Geometry: final body of the model. Coordinates: model frame, mm. A direction names the side the tool comes from. Give positions to 0.01 mm unless a question says otherwise; leave off trailing zeros. Write each loop counter-clockwise with the first axis right and the second up, starting at its lowest first coordinate (ties: lowest second). Pieces come first, ordered by that corner, then holes. Notation, with made-up numbers: M 78.25,28 L 133.25,28 A22 ccw 133.25,53 Z; hole C 69.25,-16.5 d9. An arc over 180 degrees is marked long. Use a Markdown table: item, result. Add a question column.
1) Pin query (flat end, axial travel): pin 1 (0.9 mm diameter, centred on x = 59, z = 5, fed in from +Y); pin 2 (2.5 mm diameter, centred on x = 29.5, y = 31, fed in from -Z); pin 3 (1 mm diameter, centred on x = -60.5, z = 1, fed in from -Y); pin 4 (2.5 mm diameter, centred on x = 56.5, z = 4.5, fed in from -Y). Return the tip coordinate at first contact, or that it passes through.
2) Section D-D on z = 4. State how many separate pieces and enclosed holes the cut face has, then the cut area to 3 significant figures.
3) Section A-A on y = 9. Return the cut outline in (x, z) (3 decimals), then the cut area to 3 significant figures.
4) Section B-B on y = 1. Return the cut outline in (x, z) (3 decimals).
5) Line query: line 1 (X direction, y = 5.5, z = 4.75) (3 decimals); line 2 (X direction, y = 29, z = 2.25) (3 decimals); line 3 (Z direction, x = 22, y = 11.5). Output: solid intervals per line, ascending.
6) Set-up query: faces 1 (the flat face through (13, 30, 2.75)), 2 (the flat face through (14.531, 12.6, 2.6)), 3 (the flat face through (21.175, 28, 4)). Return all of +Z, -Z, +X, -X, +Y, -Y with unobstructed straight access to the full face (end or side cutting, diameter ignored); none if empty.
7) Section C-C on x = 26.5. Return the cut outline in (y, z), then the cut area to 3 significant figures.
8) Draft query along X for faces 4 (the flat face through (46, 30, 2.75)), 5 (the flat face through (19, 4.871, 4)), 6 (the flat face through (62.175, -11.7, 2.6)). Return one class per face: +X half, -X half, draft (parallel to the pull), parting line (faces both ways), or undercut.
```python
from build123d import *

# Parameters (mm, degrees)
F0_R          = 2.5
F1_DEPTH      = 2
F3_R          = 0.99999
F2_W          = 15.5
F2_H          = 9
F2_W_2        = 9
F2_H_2        = 15.5
F2_W_3        = 37
F2_H_3        = 37
F4_DEPTH      = 0.5
F5_DEPTH      = 0.5
F6_DEPTH      = 5
F7_W          = 14
F7_H          = 3
F8_DEPTH      = 107.3565227488
F8_DEPTH_BACK = 60.2954772512
F9_W          = 13
F9_H          = 3
F10_DEPTH     = 5
F11_DEPTH     = 4


# Not quite as in the source:
# - a fillet or chamfer is up to 0.001 mm smaller than in the source, because OpenCascade refuses the exact size


with BuildPart() as f1:
    # F0 (on Top) → F1 (new body)
    with BuildSketch(Plane.XY):
        Polygon((83.825, -24.3705166107), (83.825, 32.3705166107), (-83.825, 32.3705166107), (-83.825, -32.3705166107), (-68.825, -32.3705166107), (-68.825, -24.3705166107), (-50.825, -24.3705166107), (-50.825, -32.3705166107), (-42.825, -32.3705166107), (-42.825, -24.3705166107), (-38.825, -24.3705166107), (-38.825, -36.5294833893), (-27.825, -36.5294833893), (-27.825, -28.5294833893), (-25.825, -28.5294833893), (-25.825, -36.5294833893), (45.175, -36.5294833893), (45.175, -24.3705166107), align=None)
        with Locations((-76.325, -27.6294833893)):
            Circle(F0_R, mode=Mode.SUBTRACT)
        with Locations((-76.325, 15.8705166107)):
            Circle(F0_R, mode=Mode.SUBTRACT)
    extrude(amount=F1_DEPTH)

    # F3 (radius 1 in the source; OpenCascade refuses exactly that, so slightly less here)
    f3_edges = [f1.edges().sort_by_distance(p)[0] for p in [
        (-83.825, -32.370517, 1),
        (-68.825, -32.370517, 1),
        (-68.825, -24.370517, 1),
        (-50.825, -32.370517, 1),
        (-42.825, -32.370517, 1),
        (-42.825, -24.370517, 1),
        (-38.825, -36.529483, 1),
        (-27.825, -36.529483, 1),
        (-27.825, -28.529483, 1),
        (-25.825, -36.529483, 1),
        (83.825, -24.370517, 1),
        (45.175, -24.370517, 1),
        (45.175, -36.529483, 1),
        (83.825, 32.370517, 1),
        (-83.825, 32.370517, 1),
        (-50.825, -24.370517, 1),
        (-38.825, -24.370517, 1),
        (-25.825, -28.529483, 1),
    ]]
    fillet(f3_edges, radius=F3_R)

    # F2 (on face) → F4 (cut)
    with BuildSketch(Plane.XY.offset(2)):
        with Locations((-70.075, 27.8705166107)):
            Rectangle(F2_W, F2_H)
        with Locations((-53.575, 27.8705166107)):
            Rectangle(F2_W, F2_H)
        with Locations((-37.075, 27.8705166107)):
            Rectangle(F2_W, F2_H)
        with Locations((-20.575, 27.8705166107)):
            Rectangle(F2_W, F2_H)
        with Locations((-4.075, 27.8705166107)):
            Rectangle(F2_W, F2_H)
        with Locations((12.425, 27.8705166107)):
            Rectangle(F2_W, F2_H)
        with Locations((28.925, 27.8705166107)):
            Rectangle(F2_W, F2_H)
        with Locations((45.425, 27.8705166107)):
            Rectangle(F2_W, F2_H)
        with Locations((61.925, 27.8705166107)):
            Rectangle(F2_W, F2_H)
        with Locations((57.675, 12.6205166107)):
            Rectangle(F2_W_2, F2_H_2)
        with Locations((57.675, -11.6205166107)):
            Rectangle(F2_W_2, F2_H_2)
        with Locations((19.0305227488, 12.6205166107)):
            Rectangle(F2_W_2, F2_H_2)
        with Locations((19.0305227488, -11.6205166107)):
            Rectangle(F2_W_2, F2_H_2)
        with Locations((-33.1395904124, -0.086670503)):
            Rectangle(F2_W_3, F2_H_3)
    extrude(amount=-F4_DEPTH, mode=Mode.SUBTRACT)

    # F5 (add, through all): faces of the model
    f5_faces = [f1.faces().sort_by_distance(p)[0] for p in [
        (-70.075, 27.8705166107, 1.5),
        (-53.575, 27.8705166107, 1.5),
        (-37.075, 27.8705166107, 1.5),
        (-20.575, 27.8705166107, 1.5),
        (-4.075, 27.8705166107, 1.5),
    ]]
    extrude(f5_faces, amount=F5_DEPTH)

    # F6 (add): faces of the model
    f6_faces = [f1.faces().sort_by_distance(p)[0] for p in [
        (12.425, 27.8705166107, 1.5),
        (28.925, 27.8705166107, 1.5),
        (45.425, 27.8705166107, 1.5),
        (61.925, 27.8705166107, 1.5),
        (19.0305227488, 12.6205166107, 1.5),
        (57.675, 12.6205166107, 1.5),
        (19.0305227488, -11.6205166107, 1.5),
        (57.675, -11.6205166107, 1.5),
    ]]
    extrude(f6_faces, amount=F6_DEPTH)

    # F7 (on face) → F8 (cut, two sides)
    with BuildSketch(Plane.YZ.offset(23.5305227488)) as f8_sk:
        with Locations((-11.6205166107, 4.4102044776)):
            Rectangle(F7_W, F7_H)
        with Locations((12.6205166107, 4.4102044776)):
            Rectangle(F7_W, F7_H)
    extrude(amount=-F8_DEPTH, mode=Mode.SUBTRACT)
    extrude(f8_sk.sketch, amount=F8_DEPTH_BACK, mode=Mode.SUBTRACT)

    # F9 (on face) → F10 (cut)
    with BuildSketch(Plane(origin=(0, 32.3705166107, 0), x_dir=(-1, 0, 0), z_dir=(0, 1, 0))):
        with Locations((-12.425, 4.25)):
            Rectangle(F9_W, F9_H)
        with Locations((-28.925, 4.25)):
            Rectangle(F9_W, F9_H)
        with Locations((-45.425, 4.25)):
            Rectangle(F9_W, F9_H)
        with Locations((-61.925, 4.25)):
            Rectangle(F9_W, F9_H)
    extrude(amount=-F10_DEPTH, mode=Mode.SUBTRACT)

    # F11 (add): a face of the model
    f11_faces = [f1.faces().sort_by_distance(p)[0] for p in [
        (-33.1395904124, -0.086670503, 1.5),
    ]]
    extrude(f11_faces, amount=F11_DEPTH)


solid = f1.part
```
Found:
| question | item | result |
|---|---|---|
| 1 | pin 1 | y = 27.37 |
| 1 | pin 2 | z = 0 |
| 1 | pin 3 | y = -24.37 |
| 1 | pin 4 | y = -19.37 |
| 2 | separate pieces | 13 |
| 2 | enclosed holes | 0 |
| 2 | area | 1,720 mm² |
| 3 | outline | M -83.825,0 L 83.825,0 L 83.825,2 L 62.175,2 L 62.175,2.91 L 53.175,2.91 L 53.175,2 L 23.531,2 L 23.531,2.91 L 14.531,2.91 L 14.531,2 L -14.64,2 L -14.64,5.5 L -51.64,5.5 L -51.64,2 L -83.825,2 Z; M 14.531,5.91 L 23.531,5.91 L 23.531,6.5 L 14.531,6.5 Z; M 53.175,5.91 L 62.175,5.91 L 62.175,6.5 L 53.175,6.5 Z |
| 3 | area | 492 mm² |
| 4 | outline | M -83.825,0 L 83.825,0 L 83.825,2 L -14.64,2 L -14.64,5.5 L -51.64,5.5 L -51.64,2 L -83.825,2 Z |
| 5 | line 1 | -51.64 to -14.64, 14.531 to 23.531, 53.175 to 62.175 |
| 5 | line 2 | 4.675 to 20.175, 21.175 to 36.675, 37.675 to 53.175, 54.175 to 69.675 |
| 5 | line 3 | 0 to 2.91, 5.91 to 6.5 |
| 6 | face 1 | +Y |
| 6 | face 2 | +Z, -Y |
| 6 | face 3 | +Z, +Y |
| 7 | outline | M -36.53,0 L 32.37,0 L 32.37,2.75 L 27.37,2.75 L 27.37,5.75 L 32.37,5.75 L 32.37,6.5 L 23.37,6.5 L 23.37,2 L -36.53,2 Z |
| 7 | area | 163 mm² |
| 8 | face 4 | undercut |
| 8 | face 5 | draft |
| 8 | face 6 | +X half |
